Design review of the part built by this model. Coordinates are the model's own, in mm. Face numbers are marked on the shaded views. A direction names the side the tool comes from. Coordinates: 2 decimals unless noted, no trailing zeros. Loops run counter-clockwise (first coordinate to the right, second up) from the corner with the lowest first, then second, coordinate; pieces in that order, holes last. Notation, with made-up numbers: (-15, 88.25) -> (-9, 88.25) arc R12 ccw to (-9, 110.25) -> close; hole circle Ø9 at (-17, -24). An arc over 180 degrees is marked (long way). Use one line per item in the form item = value. Start each with the question number.
1. Wall thickness on line 1 (X direction, y = 38.5, z = 45); line 2 (Y direction, x = 16.5, z = 5.5); line 3 (Z direction, x = 17.5, y = -17.5): over which ranges is each line inside the solid? List them lowest first. Write a range as from..to.
2. Consider section C-C (x = 34.5). State the section outline as (y, z) points.
3. Consider section D-D (x = 5.5). State the section outline as (y, z) points.
4. Consider section A-A (x = 19.5). State the section outline as (y, z) points, then the cut area to 3 significant figures.
5. Machinability: for the marked faces 1 and 2, which of the approach directions +Z, -Z, +X, -X, +Y, -Y give a long, thin tool a straight path to every point of the face, cutting with its end or side? Answer none if there is none.
6. Consider section B-B (y = -15). State the section outline as (x, z) points.
from build123d import *

# Parameters (mm, degrees)
F1_DEPTH = 40
F3_DEPTH = 25
F4_R     = 3
F6_DEPTH = 25


with BuildPart() as f1:
    # F0 (on Right) → F1 (new body)
    with BuildSketch(Plane.YZ):
        Polygon((-44.45, 6.35), (-44.45, 0), (44.45, 0), (44.45, 63.5), (38.1, 63.5), (38.1, 6.35), align=None)
    extrude(amount=F1_DEPTH)

    # F2 (on face) → F3 (cut)
    with BuildSketch(Plane.XY.offset(6.35)):
        with BuildLine():
            ThreePointArc((7.5, -26.45), (5.5, -24.45), (3.5, -26.45))
            ThreePointArc((3.5, -26.45), (12.4510902307, -39.8462532214), (28.2530483272, -36.7030483272))
            ThreePointArc((28.2530483272, -36.7030483272), (28.2530483272, -33.8746212025), (25.4246212025, -33.8746212025))
            ThreePointArc((25.4246212025, -33.8746212025), (13.9818239602, -36.1507350914), (7.5, -26.45))
        make_face()
        with BuildLine():
            ThreePointArc((28.5, -26.45), (30.5, -28.45), (32.5, -26.45))
            ThreePointArc((32.5, -26.45), (23.5489097693, -13.0537467786), (7.7469516728, -16.1969516728))
            ThreePointArc((7.7469516728, -16.1969516728), (7.7469516728, -19.0253787975), (10.5753787975, -19.0253787975))
            ThreePointArc((10.5753787975, -19.0253787975), (22.0181760398, -16.7492649086), (28.5, -26.45))
        make_face()
    extrude(amount=-F3_DEPTH, mode=Mode.SUBTRACT)

    # F4
    f4_edges = [f1.edges().sort_by_distance(p)[0] for p in [
        (20, 38.1, 6.35),
    ]]
    fillet(f4_edges, radius=F4_R)

    # F5 (on face) → F6 (cut)
    with BuildSketch(Plane.XZ.offset(-38.1)):
        with BuildLine():
            ThreePointArc((13.5, 53.925), (10, 57.425), (6.5, 53.925))
            Line((6.5, 53.925), (6.5, 18.925))
            ThreePointArc((6.5, 18.925), (10, 15.425), (13.5, 18.925))
            Line((13.5, 18.925), (13.5, 53.925))
        make_face()
        with BuildLine():
            ThreePointArc((33.5, 53.925), (30, 57.425), (26.5, 53.925))
            Line((26.5, 53.925), (26.5, 18.925))
            ThreePointArc((26.5, 18.925), (30, 15.425), (33.5, 18.925))
            Line((33.5, 18.925), (33.5, 53.925))
        make_face()
    extrude(amount=-F6_DEPTH, mode=Mode.SUBTRACT)


solid = f1.part
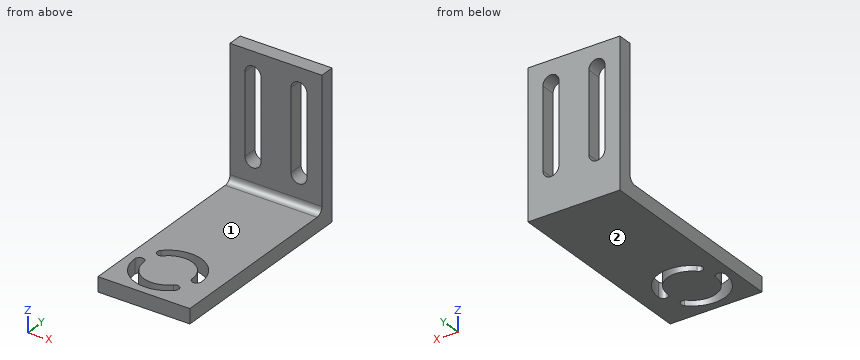
Geometry check:
q1.line_1 = 0..6.5, 13.5..26.5, 33.5..40
q1.line_2 = -44.45..-40.87, -36.84..-16.06, -12.03..44.45
q1.line_3 = 0..6.35
q2.outline = (-44.45, 0) -> (44.45, 0) -> (44.45, 63.5) -> (38.1, 63.5) -> (38.1, 9.35) arc R3 cw to (35.1, 6.35) -> (-44.45, 6.35) -> close
q3.outline = (-44.45, 0) -> (-33.8, 0) -> (-33.8, 6.35) -> (-44.45, 6.35) -> close; (-24.45, 0) -> (44.45, 0) -> (44.45, 63.5) -> (38.1, 63.5) -> (38.1, 9.35) arc R3 cw to (35.1, 6.35) -> (-24.45, 6.35) -> close
q4.outline = (-44.45, 0) -> (-40.87, 0) -> (-40.87, 6.35) -> (-44.45, 6.35) -> close; (-36.84, 0) -> (-16.06, 0) -> (-16.06, 6.35) -> (-36.84, 6.35) -> close; (-12.03, 0) -> (44.45, 0) -> (44.45, 63.5) -> (38.1, 63.5) -> (38.1, 9.35) arc R3 cw to (35.1, 6.35) -> (-12.03, 6.35) -> close
q4.area = 878 mm²
q5.face_1 = +Z, +X, -X, -Y
q5.face_2 = -Z, +X, -X, +Y, -Y
q6.outline = (0, 0) -> (9.1, 0) -> (9.1, 6.35) -> (0, 6.35) -> close; (26.9, 0) -> (40, 0) -> (40, 6.35) -> (26.9, 6.35) -> close
